Read the model definition and answer for the solid it produces. Units are mm, in the model's axes. Face numbers are marked on the shaded views. A direction names the side the tool comes from. Coordinates: 2 decimals unless noted, no trailing zeros. Loops run counter-clockwise (first coordinate to the right, second up) from the corner with the lowest first, then second, coordinate; pieces in that order, holes last. Notation, with made-up numbers: (46, -19) -> (75, -19) arc R17 ccw to (75, 14) -> close; hole circle Ø3 at (4, 83). An arc over 180 degrees is marked (long way). Answer as a JSON object with one key per item and string values. Group by question number.
1) Section A-A, the plane y = 11 is taken. Give the vertices of the cut face in (x, z), plus the area to 3 significant figures.
2) Section B-B, the plane z = 12.5 is taken. Give the vertices of the cut face in (x, y).
3) Section C-C, the plane y = -4 is taken. Give the vertices of the cut face in (x, z).
4) Section D-D, the plane x = 22.5 is taken. Give the vertices of the cut face in (y, z).
5) Consider probe 1 along Y at (x, z) = (22.5, 11.5); probe 2 along Z at (x, y) = (0, -10); probe 3 along X at (y, z) = (-19.5, 18.5). Determine where each line is inside the solid, lowest interval first. Write a range as [from, to].
6) Which of the six approach directions +Z, -Z, +X, -X, +Y, -Y give full straight-line access (tool end or side, diameter ignored) to the marked faces 1 and 2?
7) Determine the mould class of the marked faces 3, 4 and 5 for opening direction X: released by +X, released by -X, zero draft, split by the parting line, or undercut.
8) Flat-ended cylindrical pins translate along their axes: P1, Ø6.5, axis at x = 22.5, y = -11, coming from the -Z side; P2, Ø5, axis at x = 16, y = 11.5, coming from the +Z side. Find the tip coordinate at first contact, or state that the pin passes through.
from build123d import *

# Parameters (mm, degrees)
F0_W     = 25
F0_H     = 44
F1_DEPTH = 25
F2_R     = 8.5
F3_DEPTH = 44.001
F0_W_2   = 20
F0_R     = 3.5
F4_DEPTH = 20
F5_R     = 5


# Not quite as in the source:
# - a feature names something its author has since deleted; it is built from what else it names


with BuildPart() as f1:
    # F0 (on Top) → F1 (new body)
    with BuildSketch(Plane.XY):
        Rectangle(F0_W, F0_H)
    extrude(amount=F1_DEPTH)

    # F2 (on face) → F3 (cut, through all)
    with BuildSketch(Plane.XZ.offset(22)):
        with Locations((0, 12.5)):
            Circle(F2_R)
    extrude(amount=-F3_DEPTH, mode=Mode.SUBTRACT)

    # F0 (on Top) → F4 (join)
    with BuildSketch(Plane.XY):
        with Locations((22.5, 0)):
            Rectangle(F0_W_2, F0_H)
        with Locations((22.5, -11)):
            Circle(F0_R, mode=Mode.SUBTRACT)
        with Locations((22.5, 11)):
            Circle(F0_R, mode=Mode.SUBTRACT)
    extrude(amount=F4_DEPTH)

    # F5
    f5_edges = [f1.edges().sort_by_distance(p)[0] for p in [
        (-12.5, 0, 25),
        (-12.5, 0, 0),
    ]]
    fillet(f5_edges, radius=F5_R)


solid = f1.part
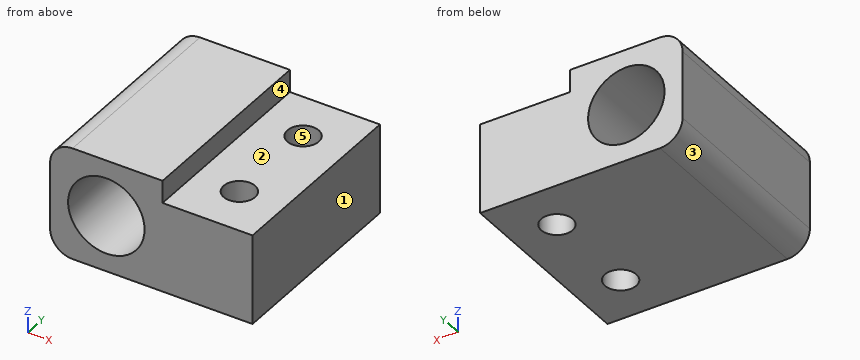
Determined:
{
 "1": {"outline": "(-12.5, 5) arc R5 ccw to (-7.5, 0) -> (19, 0) -> (19, 20) -> (12.5, 20) -> (12.5, 25) -> (-7.5, 25) arc R5 ccw to (-12.5, 20) -> close; (26, 0) -> (32.5, 0) -> (32.5, 20) -> (26, 20) -> close; hole circle Ø17 at (0, 12.5)", "area": "647 mm²"},
 "2": {"outline": "(-12.5, -22) -> (-8.5, -22) -> (-8.5, 22) -> (-12.5, 22) -> close; (8.5, -22) -> (32.5, -22) -> (32.5, 22) -> (8.5, 22) -> close; hole circle Ø7 at (22.5, -11); hole circle Ø7 at (22.5, 11)"},
 "3": {"outline": "(-12.5, 5) arc R5 ccw to (-7.5, 0) -> (32.5, 0) -> (32.5, 20) -> (12.5, 20) -> (12.5, 25) -> (-7.5, 25) arc R5 ccw to (-12.5, 20) -> close; hole circle Ø17 at (0, 12.5)"},
 "4": {"outline": "(-22, 0) -> (-14.5, 0) -> (-14.5, 20) -> (-22, 20) -> close; (-7.5, 0) -> (7.5, 0) -> (7.5, 20) -> (-7.5, 20) -> close; (14.5, 0) -> (22, 0) -> (22, 20) -> (14.5, 20) -> close"},
 "5": {"probe 1": "[-22, -14.5], [-7.5, 7.5], [14.5, 22]", "probe 2": "[0, 4], [21, 25]", "probe 3": "[-12.5, -6.02], [6.02, 32.5]"},
 "6": {"face 1": "+Z, -Z, +X, +Y, -Y", "face 2": "+Z, +X, +Y, -Y"},
 "7": {"face 3": "released by -X", "face 4": "released by +X", "face 5": "undercut"},
 "8": {"P1": "through", "P2": "z = 20"}
}
